Geometry check sheet. Reference: the model listing, model coordinates, mm. Face numbers are marked on the shaded views. A direction names the side the tool comes from. Give positions to 0.01 mm unless a question says otherwise; leave off trailing zeros. Order: outer loops, then holes, each group sorted by start corner. A loop starts at its lowest first (then second) coordinate and runs counter-clockwise, first axis right, second up.
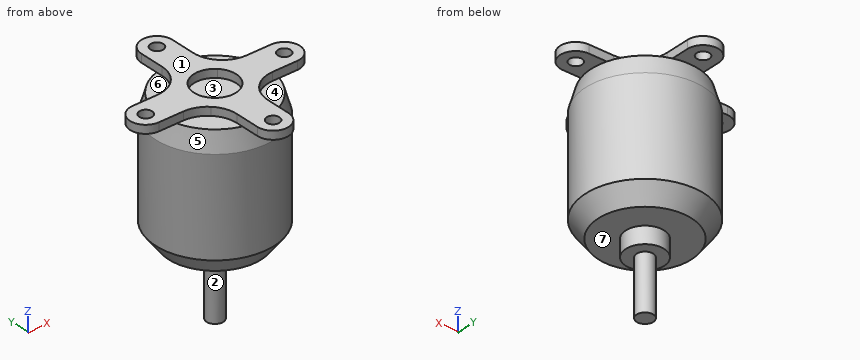
```python
from build123d import *

# Parameters (mm, degrees)
SKETCH2_R           = 1.5
BOSS_EXTRUDE1_DEPTH = 1.9304
CIRPATTERN1_COUNT   = 4


with BuildPart() as part:
    # Sketch1 → Revolve1 (revolve)
    with BuildSketch(Plane(origin=(0, 0, 0), x_dir=(0, 0, -1), z_dir=(1, 0, 0))):
        Polygon((0, 0), (0, 12.5857), (4.4704, 13.9065), (26.9748, 13.9065), (31.0388, 10.922), (31.0388, 4.50215), (34.9758, 4.50215), (34.9758, 1.9685), (47.879, 1.9685), (47.879, 0), align=None)
    revolve(axis=Axis((0, 0, 0), (0, 0, 1)))

    # Sketch2 → Boss-Extrude1 (add)
    with BuildSketch(Plane.XY):
        with BuildLine():
            Line((-3.6576, 12.04250002), (-3.6576, 10.483480973))
            Line((-3.6576, 10.483480973), (-3.6576, 3.6576))
            Line((-3.6576, 3.6576), (-3.502299887, 3.502299887))
            ThreePointArc((-3.502299887, 3.502299887), (0, 4.953), (3.502299887, 3.502299887))
            Line((3.502299887, 3.502299887), (3.6576, 3.6576))
            Line((3.6576, 3.6576), (3.6576, 10.483480973))
            Line((3.6576, 10.483480973), (3.6576, 12.04250002))
            ThreePointArc((3.6576, 12.04250002), (0, 12.5857), (-3.6576, 12.04250002))
        make_face()
        with BuildLine():
            Line((-3.6576, 3.6576), (-3.6576, 10.483480973))
            ThreePointArc((-3.6576, 10.483480973), (-4.177189251, 7.871329413), (-5.656854249, 5.656854249))
            Line((-5.656854249, 5.656854249), (-3.6576, 3.6576))
        make_face()
        with BuildLine():
            ThreePointArc((5.656854249, 5.656854249), (4.177189251, 7.871329413), (3.6576, 10.483480973))
            Line((3.6576, 10.483480973), (3.6576, 3.6576))
            Line((3.6576, 3.6576), (5.656854249, 5.656854249))
        make_face()
        with BuildLine():
            Line((-3.6576, 16.265), (-3.6576, 12.04250002))
            ThreePointArc((-3.6576, 12.04250002), (0, 12.5857), (3.6576, 12.04250002))
            Line((3.6576, 12.04250002), (3.6576, 16.265))
            ThreePointArc((3.6576, 16.265), (0, 19.9226), (-3.6576, 16.265))
        make_face()
        with Locations((0, 16.265)):
            Circle(SKETCH2_R, mode=Mode.SUBTRACT)
    boss_extrude1 = extrude(amount=BOSS_EXTRUDE1_DEPTH)

    # CirPattern1: Boss-Extrude1 ×4 about axis
    cirpattern1_axis = Axis((0, 0, 0), (0, 0, 1))
    for i in range(1, CIRPATTERN1_COUNT):
        add(boss_extrude1.rotate(cirpattern1_axis, i * 360 / CIRPATTERN1_COUNT))


solid = part.part
```
Q1. Thickness scan on L1, parallel to X at y = 0, z = 1.2 (3 decimals); L2, parallel to Z at x = 4, y = 3.5; L3, parallel to Z at x = 1.5, y = 2. Record the ranges inside material, lowest first.
Q2. Cross-section at D-D, the plane z = -38.5. Record the boundary of the cut face in (x, y), and give its area (3 significant figures).
Q3. Cross-section at C-C, the plane z = -10. Record the boundary of the cut face in (x, y).
Q4. Access from +Z, -Z, +X, -X, +Y, -Y to the whole of each face (thin tool, end or side, straight path). Record for the marked faces 4, 5, 6 and 7.
Q5. Cross-section at A-A, the plane y = 0. Give the number of separate pieces and of enclosed holes in the cut face, and give its area (3 significant figures).
Q6. Gauge pin test, flat ends, axial feed: P1, Ø8, axis at x = -10, z = -33, coming from the +Y side; P2, Ø4, axis at x = 14, y = -1.5, coming from the -Z side; P3, Ø4, axis at y = -10.5, z = -9, coming from the -X side. Record the tip position at first contact, or that the pin passes through.
Q7. Release check for a two-part mould opening along X. For the marked faces 1, 2 and 3 record: pulls with the +X half, pulls with the -X half, needs draft (parallel to the pull), parting line crosses it, or undercut.
Answers follow:
1. L1: x = -19.923 to -17.765, -14.765 to -4.953, 4.953 to 14.765, 17.765 to 19.923
1. L2: z = -31.04 to 1.93
1. L3: z = -34.98 to 0
2. outline: circle Ø3.94 at (0, 0)
2. area: 12.2 mm2
3. outline: circle Ø27.81 at (0, 0)
4. face 4: +Z, +X, -Y
4. face 5: none
4. face 6: +Z, -X, +Y
4. face 7: -Z
5. separate pieces: 3
5. enclosed holes: 0
5. area: 978 mm2
6. P1: stops at y = 9.08
6. P2: stops at z = -29.46
6. P3: stops at x = -11.01
7. face 1: needs draft
7. face 2: parting line crosses it
7. face 3: undercut
